```python
from build123d import *

# Parameters (mm, degrees)
SKETCH_4_W          = 16
SKETCH_4_H          = 27.3
EXTRUDE_3_DEPTH     = 45
SHELL_2_OUTLINE_R   = 31.1
SHELL_2_OUTLINE_R_2 = 9
SHELL_2_DEPTH       = 89
SHELL_START         = 63.7
SHELL_2_2_DEPTH     = 25.3
SHELL_2_3_OUTLINE_R = 9
SHELL_2_3_DEPTH     = 19


# Read off the part's stored shape, not the designer's step: 쉘2
with BuildPart() as part:
    # 스케치3 → 회전1 (revolve)
    with BuildSketch(Plane.XY, mode=Mode.PRIVATE) as revolve_1_sk:
        Polygon((0, 19), (8, 19), (8, 90), (32.1, 90), (32.1, 0), (0, 0), align=None)
    revolve(revolve_1_sk.sketch.rotate(Axis((0, 0, 0), (0, 1, 0)), 90), axis=Axis((0, 0, 0), (0, 1, 0)))

    # 스케치4 → 보스-돌출3 (add)
    with BuildSketch(Plane.XY):
        with Locations((-24.1, 76.35)):
            Rectangle(SKETCH_4_W, SKETCH_4_H)
    extrude(amount=EXTRUDE_3_DEPTH)

    # 쉘2 outline → 쉘2 (cut)
    with BuildSketch(Plane(origin=(0, 0, 0), x_dir=(1, 0, 0), z_dir=(0, 1, 0))):
        Circle(SHELL_2_OUTLINE_R)
        Circle(SHELL_2_OUTLINE_R_2, mode=Mode.SUBTRACT)
    extrude(amount=SHELL_2_DEPTH, mode=Mode.SUBTRACT)

    # Shell 2 2 outline → Shell 2 2 (cut)
    with BuildSketch(Plane(origin=(0, 0, 0), x_dir=(1, 0, 0), z_dir=(0, 1, 0)).offset(SHELL_START)):
        with BuildLine():
            ThreePointArc((-17.1, -25.976912827), (-27.377180278, -14.754660281), (-31.1, 0))
            Line((-31.1, 0), (-31.1, -45))
            Line((-31.1, -45), (-17.1, -45))
            Line((-17.1, -45), (-17.1, -25.976912827))
        make_face()
    extrude(amount=SHELL_2_2_DEPTH, mode=Mode.SUBTRACT)

    # Shell 2 3 outline → Shell 2 3 (cut)
    with BuildSketch(Plane(origin=(0, 0, 0), x_dir=(1, 0, 0), z_dir=(0, 1, 0))):
        Circle(SHELL_2_3_OUTLINE_R)
    extrude(amount=SHELL_2_3_DEPTH, mode=Mode.SUBTRACT)


solid = part.part
```
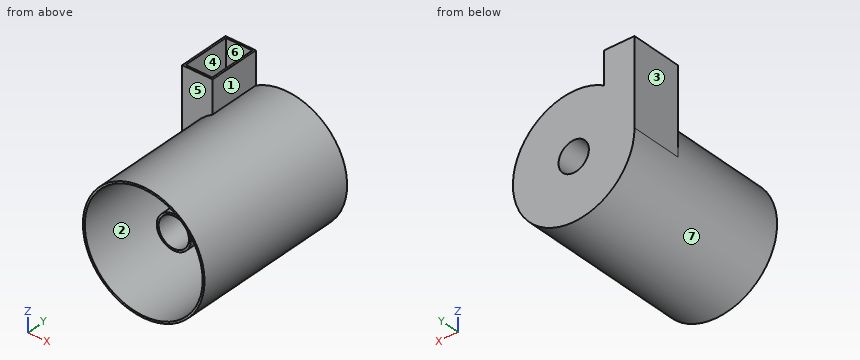
CAD build for the part. Positions are in the model's coordinates, mm. Face numbers are marked on the shaded views. A direction names the side the tool comes from. Give positions to 0.01 mm unless a question says otherwise; leave off trailing zeros. Order: outer loops, then holes, each group sorted by start corner. A loop starts at its lowest first (then second) coordinate and runs counter-clockwise, first axis right, second up. Notation, with made-up numbers: M 83,64.5 L 99,64.5 A12 cw 99,70.5 Z; hole C -23,76.5 d11. An arc over 180 degrees is marked long. Put each result on its own line as item: value. Start each with the question number.
(1) Saw through at A-A, the plane y = 79. Write the cut outline in (x, z), then the cut area to 3 significant figures.
(2) Mould opens along Y. For the marked faces 5, 6 and 7 say: +Y half, -Y half, draft (parallel to the pull), parting line (faces both ways), or undercut.
(3) Saw through at C-C, the plane z = -1.5. Write the cut outline in (x, y).
(4) Drill centre lines: line 1 along X through (y, z) = (51, 0); line 2 along X through (y, z) = (66.5, 33.5); line 3 along Z through (x, y) = (2.5, 79). Where is each one in solid material? Low to high.
(5) Which spindle directions (+Z, -Z, +X, -X, +Y, -Y) get a long thin tool onto all of the face, cutting with end or side? Do the marked faces 1, 2, 3 and 4. Say none if no direction does.
(6) Saw through at D-D, the plane y = 61.5. Write the cut outline in (x, z), then the cut area to 3 significant figures.
(7) Saw through at B-B, the plane x = 0. Write the cut outline in (y, z), then the cut area to 3 significant figures.
(8) Flat gauge pins, fed straight in: pin 1 Ø1.5 at (x, y) = (9, 25) entering from -Z; pin 2 Ø8 at (x, z) = (-3.5, -1.5) entering from +Y; pin 3 Ø4 at (y, z) = (18, 31.5) entering from +X; pin 4 Ø12 at (x, y) = (-19, 80.5) entering from -Z. Where does each tip first touch, or does it go through?
Check result:
1. outline: M -32.1,0 A32.1 ccw long -16.1,27.77 L -16.1,45 L -17.1,45 L -17.1,25.98 A31.1 cw long -31.1,0 L -31.1,45 L -32.1,45 Z; C 0,0 d18; hole C 0,0 d16
1. area: 283 mm2
2. face 5: -Y half
2. face 6: undercut
2. face 7: draft
3. outline: M -32.06,0 L -31.06,0 L -31.06,89 L -8.87,89 L -8.87,19 L -7.86,19 L -7.86,90 L -32.06,90 Z; M 7.86,19 L 8.87,19 L 8.87,89 L 31.06,89 L 31.06,0 L 32.06,0 L 32.06,90 L 7.86,90 Z
4. line 1: x = -32.1 to -31.1, -9 to -8, 8 to 9, 31.1 to 32.1
4. line 2: x = -32.1 to -31.1, -17.1 to -16.1
4. line 3: z = -32 to -31, -8.65 to -7.6, 7.6 to 8.65, 31 to 32
5. face 1: +Z, +Y, -Y
5. face 2: -Y
5. face 3: +Z, -Z, -X, +Y, -Y
5. face 4: +Z
6. outline: C 0,0 d64.2; C 0,0 d18; hole C 0,0 d62.2; hole C 0,0 d16
6. area: 252 mm2
7. outline: M 0,-32.1 L 90,-32.1 L 90,-8 L 19,-8 L 19,-9 L 89,-9 L 89,-31.1 L 0,-31.1 Z; M 0,31.1 L 89,31.1 L 89,9 L 19,9 L 19,8 L 90,8 L 90,32.1 L 0,32.1 Z
7. area: 366 mm2
8. pin 1: stops at z = -31.02
8. pin 2: passes through
8. pin 3: stops at x = 12.66
8. pin 4: stops at z = -29.35
